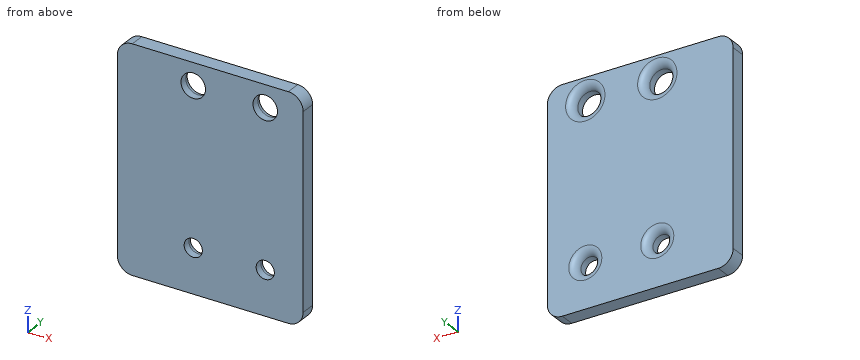
```python
from build123d import *

# Parameters (mm, degrees)
SKETCH2_W           = 25
SKETCH2_H           = 30
SKETCH2_R           = 1.225
SKETCH2_R_2         = 1.65
BOSS_EXTRUDE2_DEPTH = 2
FILLET1_R           = 2
FILLET2_R           = 1


with BuildPart() as part:
    # Sketch2 → Boss-Extrude2 (new body)
    with BuildSketch(Plane(origin=(0, 0, 0), x_dir=(1, 0, 0), z_dir=(0, 1, 0))):
        with Locations((12.5, 15)):
            Rectangle(SKETCH2_W, SKETCH2_H)
        with Locations(Location((19.9, 24, 0), (0, 0, 270))):
            Circle(SKETCH2_R, mode=Mode.SUBTRACT)
        with Locations(Location((10.21, 24, 0), (0, 0, 270))):
            Circle(SKETCH2_R, mode=Mode.SUBTRACT)
        with Locations(Location((10.21, 3, 0), (0, 0, 270))):
            Circle(SKETCH2_R_2, mode=Mode.SUBTRACT)
        with Locations(Location((19.9, 3, 0), (0, 0, 270))):
            Circle(SKETCH2_R_2, mode=Mode.SUBTRACT)
    extrude(amount=BOSS_EXTRUDE2_DEPTH)

    # Fillet1
    fillet1_edges = [part.edges().sort_by_distance(p)[0] for p in [
        (0, 1, -30),
        (25, 1, -30),
        (25, 1, 0),
        (0, 1, 0),
    ]]
    fillet(fillet1_edges, radius=FILLET1_R)

    # Fillet2
    fillet2_edges = [part.edges().sort_by_distance(p)[0] for p in [
        (19.9, 2, -25.225),
        (10.21, 2, -25.225),
        (10.21, 2, -4.65),
        (19.9, 2, -4.65),
    ]]
    fillet(fillet2_edges, radius=FILLET2_R)


solid = part.part
```
Could you check a few things on this model? Use its own coordinates, in mm. Coordinates: 2 decimals unless noted, no trailing zeros. Loops run counter-clockwise (first coordinate to the right, second up) from the corner with the lowest first, then second, coordinate; pieces in that order, holes last. Notation, with made-up numbers: M 66.25,-36.75 L 78.25,-36.75 A17 ccw 78.25,-8.75 Z; hole C 74,-10.5 d8. An arc over 180 degrees is marked long. Put each result on its own line as item: value. Start each with the question number.
(1) Suppose I cut it at A-A on z = -24. Please give me the cut outline in (x, y) (3 decimals).
(2) Will these pins go through, and if not, where does the flat tip stop? P1, Ø2.5, axis at x = 19.9, z = -3, coming from the -Y side; P2, Ø3, axis at x = 19.9, z = -24, coming from the +Y side.
(3) I need wall thicknesses on line 1 (X direction, y = 0.25, z = -3); line 2 (X direction, y = 0.45, z = -24) (3 decimals); line 3 (Z direction, x = 9.25, y = 0.55). Which ranges of each line are inside material? Lowest first, please. Write a range as from..to.
(4) Suppose I cut it at C-C on x = 10.21. Please give me the cut outline in (y, z) (3 decimals).
(5) Suppose I cut it at B-B on y = 0.45. Please give me the cut outline in (x, z) (3 decimals), then the cut area to 3 significant figures.
Solutions:
1. outline: M 0,0 L 8.985,0 L 8.985,1 A1 ccw 7.985,2 L 0,2 Z; M 11.435,0 L 18.675,0 L 18.675,1 A1 ccw 17.675,2 L 12.435,2 A1 ccw 11.435,1 Z; M 21.125,0 L 25,0 L 25,2 L 22.125,2 A1 ccw 21.125,1 Z
2. P1: passes through
2. P2: stops at y = 1.69
3. line 1: x = 0..8.56, 11.86..18.25, 21.55..25
3. line 2: x = 0..8.985, 11.435..18.675, 21.125..25
3. line 3: z = -30..-24.76, -23.24..-4.34, -1.66..0
4. outline: M 0,-30 L 2,-30 L 2,-26.225 A1 ccw 1,-25.225 L 0,-25.225 Z; M 0,-22.775 L 1,-22.775 A1 ccw 2,-21.775 L 2,-5.65 A1 ccw 1,-4.65 L 0,-4.65 Z; M 0,-1.35 L 1,-1.35 A1 ccw 2,-0.35 L 2,0 L 0,0 Z
5. outline: M 0,-28 A2 ccw 2,-30 L 23,-30 A2 ccw 25,-28 L 25,-2 A2 ccw 23,0 L 2,0 A2 ccw 0,-2 Z; hole C 10.21,-3 d3.3; hole C 10.21,-24 d2.45; hole C 19.9,-3 d3.3; hole C 19.9,-24 d2.45
5. area: 720 mm2
